```python
from build123d import *

# Parameters (mm, degrees)
SKETCH1_W           = 1000
SKETCH1_H           = 1000
BOSS_EXTRUDE2_DEPTH = 300
SKETCH1_4_W         = 155
SKETCH1_4_H         = 930
BOSS_EXTRUDE3_DEPTH = 70
SKETCH1_5_W         = 620
SKETCH1_5_H         = 930
BOSS_EXTRUDE4_DEPTH = 40


with BuildPart() as part:
    # Sketch1 → Boss-Extrude2 (new body)
    with BuildSketch(Plane(origin=(0, 0, 0), x_dir=(1, 0, 0), z_dir=(0, 1, 0))):
        Rectangle(SKETCH1_W, SKETCH1_H)
        Polygon((465, 465), (310, 465), (-310, 465), (-465, 465), (-465, -465), (-310, -465), (310, -465), (465, -465), align=None, mode=Mode.SUBTRACT)
    extrude(amount=BOSS_EXTRUDE2_DEPTH)

    # Sketch1_4 → Boss-Extrude3 (add)
    with BuildSketch(Plane(origin=(0, 0, 0), x_dir=(1, 0, 0), z_dir=(0, 1, 0))):
        with Locations((-387.5, 0)):
            Rectangle(SKETCH1_4_W, SKETCH1_4_H)
        with Locations((387.5, 0)):
            Rectangle(SKETCH1_4_W, SKETCH1_4_H)
    extrude(amount=BOSS_EXTRUDE3_DEPTH)

    # Sketch1_5 → Boss-Extrude4 (add)
    with BuildSketch(Plane(origin=(0, 0, 0), x_dir=(1, 0, 0), z_dir=(0, 1, 0))):
        Rectangle(SKETCH1_5_W, SKETCH1_5_H)
    extrude(amount=BOSS_EXTRUDE4_DEPTH)


solid = part.part
```
Geometry check sheet. Reference: the model listing, model coordinates, mm. A direction names the side the tool comes from. Round coordinates to 2 decimals unless told otherwise and drop trailing zeros. Order: outer loops, then holes, each group sorted by start corner. A loop starts at its lowest first (then second) coordinate and runs counter-clockwise, first axis right, second up. Notation, with made-up numbers: M 33.5,-21 L 48.5,-21 A31 cw 48.5,9 Z; hole C 36,-13.5 d4. An arc over 180 degrees is marked long. Answer as CSV lines item,"result".
1) Gauge pin test, flat end, axial feed: pin 1 Ø6 at (x, z) = (235.5, -272.5) entering from +Y. Record the tip position at first contact, or that the pin passes through.
Entries:
pin 1,"y = 40"
2) Mould release check, pull along Z, two halves, no side actions. Record for faces 3 (the face through (-7, 148, 500)), 4 (the face through (465, 183, 7)), 5 (the face through (-39, 300, 479)), 6 (the face through (-7, 148, -500)): +Z half, -Z half, draft (parallel to the pull), parting line (faces both ways), or undercut.
Entries:
face 3,"+Z half"
face 4,"undercut"
face 5,"draft"
face 6,"-Z half"
3) Thickness scan on probe 1 along X at (y, z) = (156, 322.5); probe 2 along X at (y, z) = (53, 51). Record the ranges inside material, lowest first. Write a range as [from, to].
Entries:
probe 1,"[-500, -465], [465, 500]"
probe 2,"[-500, -310], [310, 500]"
4) Sectioned sample at D-D on y = 279. Record the cut outline in (x, z).
Entries:
outline,"M -500,-500 L 500,-500 L 500,500 L -500,500 Z; hole M -465,-465 L 465,-465 L 465,465 L -465,465 Z"
5) Sectioned sample at A-A on y = 58. Record the cut outline in (x, z), and give its area (3 significant figures).
Entries:
outline,"M -500,-500 L 500,-500 L 500,500 L -500,500 Z; hole M -310,-465 L 310,-465 L 310,465 L -310,465 Z"
area,"423,000 mm2"
6) Sectioned sample at B-B on z = -379.5. Record the cut outline in (x, y), and give its area (3 significant figures).
Entries:
outline,"M -500,0 L 500,0 L 500,300 L 465,300 L 465,70 L 310,70 L 310,40 L -310,40 L -310,70 L -465,70 L -465,300 L -500,300 Z"
area,"67,500 mm2"
7) Sectioned sample at C-C on x = 406.5. Record the cut outline in (y, z).
Entries:
outline,"M 0,-500 L 300,-500 L 300,-465 L 70,-465 L 70,465 L 300,465 L 300,500 L 0,500 Z"
8) Tool access check on faces 1 (the face through (-500, 148, 7)), 2 (the face through (-465, 183, -7)). Record the directions out of +Z, -Z, +X, -X, +Y, -Y that give a thin tool (end or side, any length) a straight path to the whole face; none if there is none.
Entries:
face 1,"+Z, -Z, -X, +Y, -Y"
face 2,"+Y"
